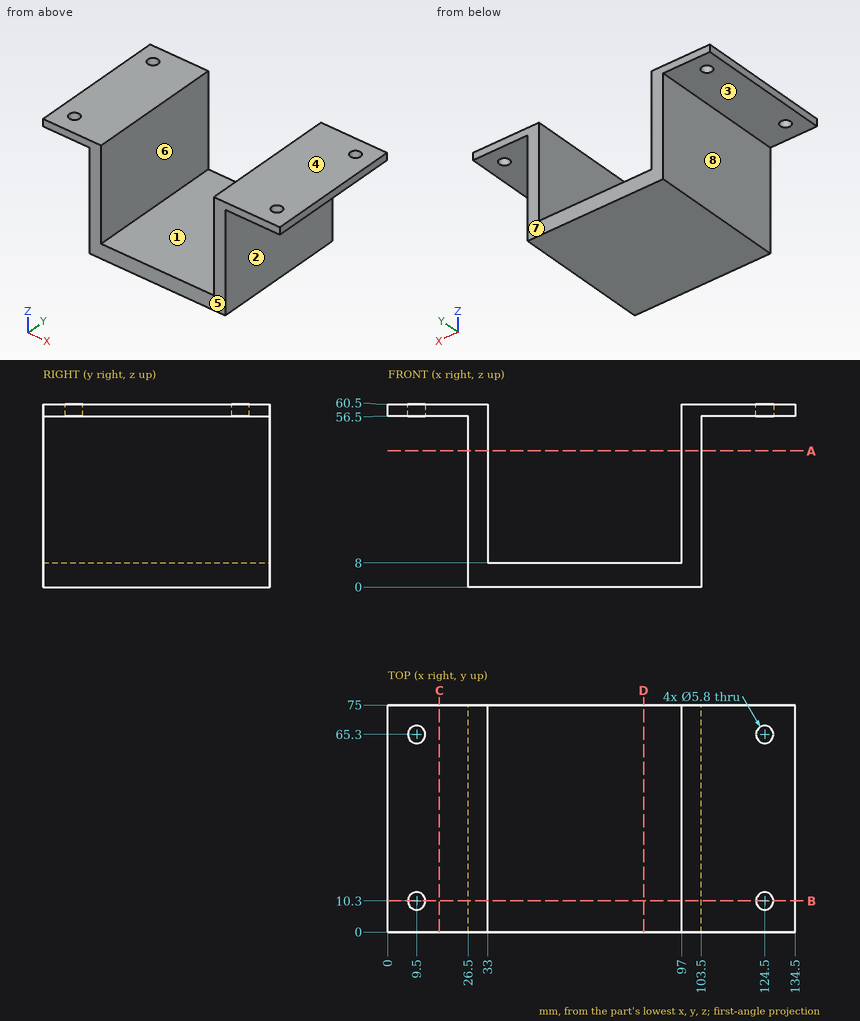
Study the drawing (mm; zero at the part's minimum x, y, z) and answer. A direction names the side the tool comes from. Coordinates: 2 decimals unless noted, no trailing zeros. Write each loop counter-clockwise with the first axis right and the second up, starting at its lowest first coordinate (ties: lowest second). Pieces come first, ordered by that corner, then holes. Notation, with made-up numbers: M -0.5,45 L 50.5,45 A13 ccw 50.5,53 Z; hole C -37,65 d5. An arc over 180 degrees is marked long. Use one line per item in the form item = value.
Item 1: Find the intervals of material crossed by probe 1 along X at (y, z) = (65, 57); probe 2 along X at (y, z) = (48.5, 47); probe 3 along Z at (x, y) = (127.5, 26), in increasing order.
Model answer:
probe_1 = 0 to 6.62, 12.38 to 33, 97 to 121.62, 127.38 to 134.5
probe_2 = 26.5 to 33, 97 to 103.5
probe_3 = 56.5 to 60.5
Item 2: Find section D-D, the plane x = 84.5. Give the vertices of the cut face in (y, z).
Model answer:
outline = M 0,0 L 75,0 L 75,8 L 0,8 Z
Item 3: Find section B-B, the plane y = 10.3. Give the vertices of the cut face in (x, z), plus the area to 3 significant figures.
Model answer:
outline = M 0,56.5 L 6.6,56.5 L 6.6,60.5 L 0,60.5 Z; M 12.4,56.5 L 26.5,56.5 L 26.5,0 L 103.5,0 L 103.5,56.5 L 121.6,56.5 L 121.6,60.5 L 97,60.5 L 97,8 L 33,8 L 33,60.5 L 12.4,60.5 Z; M 127.4,56.5 L 134.5,56.5 L 134.5,60.5 L 127.4,60.5 Z
area = 1,480 mm2
Item 4: For the marked faces 1, 2, 3, 4 and 5, determine the directions among +Z, -Z, +X, -X, +Y, -Y from which every point of the face is accessible in a straight line to the end or side of a thin tool.
Model answer:
face_1 = +Z, +Y, -Y
face_2 = -Z, +X, +Y, -Y
face_3 = -Z, -X, +Y, -Y
face_4 = +Z, +X, -X, +Y, -Y
face_5 = +Z, -Z, +X, -X, -Y
Item 5: Find section A-A, the plane z = 45. Give the vertices of the cut face in (x, y).
Model answer:
outline = M 26.5,0 L 33,0 L 33,75 L 26.5,75 Z; M 97,0 L 103.5,0 L 103.5,75 L 97,75 Z
Item 6: Given P1, Ø8, axis at y = 36, z = 42.5, coming from the +X side; P2, Ø9.5, axis at x = 9.5, y = 10.3, coming from the +Z side; P3, Ø6, axis at x = 47, y = 58.5, coming from the +Z side; P4, Ø6, axis at y = 13.5, z = 47, coming from the -X side, each flat-ended and moving along its own axis, determine where each tip first touches the part or whether it passes through.
Model answer:
P1 = 103.5
P2 = 60.5
P3 = 8
P4 = 26.5
Item 7: The mould has two halves that part along X. Classify the marked faces 6, 7 and 8: released by +X, released by -X, zero draft, split by the parting line, or undercut.
Model answer:
face_6 = undercut
face_7 = zero draft
face_8 = released by -X
Item 8: Find section C-C, the plane x = 17. Give the vertices of the cut face in (y, z).
Model answer:
outline = M 0,56.5 L 75,56.5 L 75,60.5 L 0,60.5 Z
